from build123d import *

# Parameters (mm, degrees)
FILLET_1_R          = 0.5
FILLET_2_R          = 0.5
FILLET_3_R          = 1
FILLET_4_R          = 0.5
CHAMFER_1_SIZE      = 1
CHAMFER_2_SIZE      = 1
CUT_EXTRUDE_1_DEPTH = 6


with BuildPart() as part:
    # Эскиз1 → Повернуть1 (revolve)
    with BuildSketch(Plane(origin=(0, 0, 0), x_dir=(1, 0, 0), z_dir=(0, 1, 0)), mode=Mode.PRIVATE) as revolve_1_sk:
        with BuildLine():
            Line((55.756411679, -2.497269463), (55.756411679, -6.997269463))
            Line((55.756411679, -6.997269463), (43.756411679, -6.997269463))
            Line((43.756411679, -6.997269463), (43.756411679, -8.497269463))
            Line((43.756411679, -8.497269463), (38.756411679, -8.497269463))
            Line((38.756411679, -8.497269463), (38.756411679, -10.497269463))
            Line((38.756411679, -10.497269463), (35.756411679, -10.497269463))
            Line((35.756411679, -10.497269463), (35.756411679, -8.497269463))
            Line((35.756411679, -8.497269463), (20.756411679, -8.497269463))
            ThreePointArc((20.756411679, -8.497269463), (20.229203885, -7.224477257), (18.956411679, -6.697269463))
            Line((18.956411679, -6.697269463), (16.956411679, -6.697269463))
            Line((16.956411679, -6.697269463), (15.895751507, -7.757929635))
            Line((15.895751507, -7.757929635), (-119.089435131, -7.757929635))
            Line((-119.089435131, -7.757929635), (-119.089435131, -5.757929635))
            Line((-119.089435131, -5.757929635), (-124.089435131, -5.757929635))
            Line((-124.089435131, -5.757929635), (-124.089435131, -2.497269463))
            Line((-124.089435131, -2.497269463), (55.756411679, -2.497269463))
        make_face()
    revolve(revolve_1_sk.sketch.rotate(Axis((55.756411679, 0, 2.497269463), (-1, 0, 0)), 180), axis=Axis((55.756411679, 0, 2.497269463), (-1, 0, 0)))

    # Скругление1
    fillet_1_edges = [part.edges().sort_by_distance(p)[0] for p in [
        (35.756411679, 0, 8.497269463),
    ]]
    fillet(fillet_1_edges, radius=FILLET_1_R)

    # Скругление2
    fillet_2_edges = [part.edges().sort_by_distance(p)[0] for p in [
        (38.756411679, 0, 8.497269463),
    ]]
    fillet(fillet_2_edges, radius=FILLET_2_R)

    # Скругление3
    fillet_3_edges = [part.edges().sort_by_distance(p)[0] for p in [
        (16.956411679, 0, 6.697269463),
    ]]
    fillet(fillet_3_edges, radius=FILLET_3_R)

    # Скругление4
    fillet_4_edges = [part.edges().sort_by_distance(p)[0] for p in [
        (-119.089435131, 0, 5.757929635),
    ]]
    fillet(fillet_4_edges, radius=FILLET_4_R)

    # Фаска1
    chamfer_1_edges = [part.edges().sort_by_distance(p)[0] for p in [
        (55.756411679, 0, 6.997269463),
        (-119.089435131, 0, 7.757929635),
    ]]
    chamfer(chamfer_1_edges, length=CHAMFER_1_SIZE)

    # Фаска2
    chamfer_2_edges = [part.edges().sort_by_distance(p)[0] for p in [
        (-124.089435131, 0, 5.757929635),
    ]]
    chamfer(chamfer_2_edges, length=CHAMFER_2_SIZE)

    # Эскиз2 → Вырез-Вытянуть1 (cut)
    with BuildSketch(Plane(origin=(0, 10, 0), x_dir=(1, 0, 0), z_dir=(0, 1, 0))):
        with BuildLine():
            Line((23.550856254, -0.902866319), (28.868398961, -0.902866319))
            ThreePointArc((28.868398961, -0.902866319), (30.462802104, -2.497269463), (28.868398961, -4.091672607))
            Line((28.868398961, -4.091672607), (23.550856254, -4.091672607))
            ThreePointArc((23.550856254, -4.091672607), (21.95645311, -2.497269463), (23.550856254, -0.902866319))
        make_face()
    extrude(amount=-CUT_EXTRUDE_1_DEPTH, mode=Mode.SUBTRACT)


solid = part.part
Can you work these out from the model? Positions are in its coordinate system, mm. A direction names the side the tool comes from. Coordinates: 2 decimals unless noted, no trailing zeros. Loops run counter-clockwise (first coordinate to the right, second up) from the corner with the lowest first, then second, coordinate; pieces in that order, holes last. Notation, with made-up numbers: M 51.5,88 L 64.5,88 A21 ccw 64.5,94 Z; hole C -1.75,39 d8. An arc over 180 degrees is marked long. Answer as CSV lines item,"result". Start each with the question number.
1. Suppose I cut it at A-A, the plane x = 7.5. List the corners of the cut face in (y, z) for me.
2. For pin 1 Ø1.4 at (x, y) = (27.5, 4.5) entering from +Z; pin 2 Ø1 at (y, z) = (-6, 3) entering from +X; pin 3 Ø2 at (x, y) = (26.5, 4.5) entering from -Z, each with a flat end and sliding along its axis, tell me the tip position at first contact or that it passes through.
3. For faces 1 (the face through (-119.089, 4, 3)), 2 (the face through (43.756, -4, 5)), 3 (the face through (18.15, -1.26, -1.51)), which set-ups out of +Z, -Z, +X, -X, +Y, -Y let a thin tool reach every point of the face, with its end or its side?
4. If I drill on probe 1 along Z at (x, y) = (-93.5, -0.5); probe 2 along X at (y, z) = (-6.75, 4.25); probe 3 along X at (y, z) = (5.5, 2.75), over which ranges is the centre line in solid material (lowest first)? Write a range as [from, to].
5. Thinking about a two-plate mould opening in Z: for faces 4 (the face through (-121.364, -2.204, 4.901)), 5 (the face through (26, 4, 2)), 6 (the face through (-124.089, 0, 3)), which applies, +Z half, -Z half, draft (parallel to the pull), parting line (faces both ways), or undercut?
Output:
1,outline,"C 0,2.5 d10.52"
2,pin 1,"stops at z = 7.14"
2,pin 2,"stops at x = 43.76"
2,pin 3,"stops at z = -2.38"
3,face 1,"-X"
3,face 2,"+X"
3,face 3,"none"
4,probe 1,"z = [-2.74, 7.73]"
4,probe 2,"x = [35.76, 38.76]"
4,probe 3,"x = [20.69, 21.98], [30.44, 43.76]"
5,face 4,"parting line"
5,face 5,"undercut"
5,face 6,"draft"
